```python
from build123d import *

# Parameters (mm, degrees)
F3_START = 1.5
F2_R     = 1.3
F3_DEPTH = 3.5


with BuildPart() as f1:
    # F0 (on Front) → F1 (revolve)
    with BuildSketch(Plane.XZ):
        Polygon((-39.5, 2), (-39.5, 0), (-22.5, 0), (-22.5, 1.5), (-25.4, 1.5), (-25.4, 5), (-34.4469576932, 5), (-34.4469576932, 2), align=None)
    revolve(axis=Axis((0, 0, 4.7885915264), (0, 0, -1)))

    # F2 (on Top) → F3 (cut)
    with BuildSketch(Plane.XY.offset(F3_START)):
        with Locations((0, 25.4)):
            Circle(F2_R)
        with Locations((-25.4, 0)):
            Circle(F2_R)
        with Locations((0, -25.4)):
            Circle(F2_R)
        with Locations((25.4, 0)):
            Circle(F2_R)
    extrude(amount=F3_DEPTH, mode=Mode.SUBTRACT)


solid = f1.part
```
Geometry: final body of the model. Coordinates: model frame, mm. A direction names the side the tool comes from. Give positions to 0.01 mm unless a question says otherwise; leave off trailing zeros. Write each loop counter-clockwise with the first axis right and the second up, starting at its lowest first coordinate (ties: lowest second). Pieces come first, ordered by that corner, then holes.
1. Reachability of faces 1 (the cylindrical face through (18.144, -17.775, 3.274)), 2 (the flat face through (2, 26, 5)) from +Z, -Z, +X, -X, +Y, -Y: full face, straight path, thin tool, end or side. Return the list, or none.
2. Section query A-A, the plane y = 0. Return loops of the section in (x, z), then the cut area to 3 significant figures.
3. Draft query along Y for faces 3 (the cylindrical face through (-18.144, 17.775, 3.274)), 4 (the cylindrical face through (4.484, 34.154, 3.479)), 5 (the flat face through (3, 35, 2)). Return one class per face: released by +Y, released by -Y, zero draft, split by the parting line, or undercut.
4. Pin query (flat end, axial travel): P1, Ø16, axis at x = -10.5, y = 10.5, coming from the +Z side; P2, Ø1.5, axis at x = -21, z = 4, coming from the -Y side. Return the tip coordinate at first contact, or that it passes through.
5. Line query: probe 1 along Y at (x, z) = (0, 0.65); probe 2 along X at (y, z) = (4, 1.45); probe 3 along X at (y, z) = (19, 3.8). Output: solid intervals per line, ascending.
6. Section query B-B, the plane z = 2.9. Return loops of the section in (x, y).
7. Section query D-D, the plane x = 29.5. Return loops of the section in (y, z).
Computed:
1. face 1: +Z
1. face 2: +Z, +X, -X, +Y, -Y
2. outline: (-39.5, 0) - (-22.5, 0) - (-22.5, 1.5) - (-26.7, 1.5) - (-26.7, 5) - (-34.45, 5) - (-34.45, 2) - (-39.5, 2) - close; (22.5, 0) - (39.5, 0) - (39.5, 2) - (34.45, 2) - (34.45, 5) - (26.7, 5) - (26.7, 1.5) - (22.5, 1.5) - close
2. area: 110 mm2
3. face 3: undercut
3. face 4: split by the parting line
3. face 5: zero draft
4. P1: stops at z = 1.5
4. P2: stops at y = -27.87
5. probe 1: y = -39.5 to -22.5, 22.5 to 39.5
5. probe 2: x = -39.3 to -22.14, 22.14 to 39.3
5. probe 3: x = -28.73 to -16.86, 16.86 to 28.73
6. outline: circle Ø68.89 at (0, 0); hole (-25.37, -1.3) arc R25.4 ccw to (-1.3, -25.37) arc R1.3 ccw (long way) to (1.3, -25.37) arc R25.4 ccw to (25.37, -1.3) arc R1.3 ccw (long way) to (25.37, 1.3) arc R25.4 ccw to (1.3, 25.37) arc R1.3 ccw (long way) to (-1.3, 25.37) arc R25.4 ccw to (-25.37, 1.3) arc R1.3 ccw (long way) to start
7. outline: (-26.27, 0) - (26.27, 0) - (26.27, 2) - (17.79, 2) - (17.79, 5) - (-17.79, 5) - (-17.79, 2) - (-26.27, 2) - close
